```python
from build123d import *

# Parameters (mm, degrees)
F1_DEPTH     = 56.134
F3_DEPTH     = 12.7
F4_T         = 6.35
F4_T3_DEPTH  = 38.1
F4_T5_DEPTH  = 38.1
F4_T8_ANGLE  = 90.000000001
F4_T10_ANGLE = 90.000000001
F4_T12_ANGLE = 90.000000001
F4_T14_ANGLE = 90.000000001


# Not quite as in the source:
# - a shell that OpenCascade refuses in one call is made with other operations: the cavity is built on its own and cut out


with BuildPart() as f1:
    # F0 (on Top) → F1 (new body)
    with BuildSketch(Plane.XY):
        with BuildLine():
            ThreePointArc((-38.1, -12.7), (-30.6605122421, -30.6605122421), (-12.7, -38.1))
            Line((-12.7, -38.1), (12.7, -38.1))
            ThreePointArc((12.7, -38.1), (30.6605122421, -30.6605122421), (38.1, -12.7))
            Line((38.1, -12.7), (38.1, 12.7))
            ThreePointArc((38.1, 12.7), (30.6605122421, 30.6605122421), (12.7, 38.1))
            Line((12.7, 38.1), (-12.7, 38.1))
            ThreePointArc((-12.7, 38.1), (-30.6605122421, 30.6605122421), (-38.1, 12.7))
            Line((-38.1, 12.7), (-38.1, -12.7))
        make_face()
    extrude(amount=F1_DEPTH)

    # F2 (on face) → F3 (join)
    with BuildSketch(Plane.XY.offset(56.134)):
        with BuildLine():
            ThreePointArc((-50.8, -38.1), (-47.0802561211, -47.0802561211), (-38.1, -50.8))
            Line((-38.1, -50.8), (38.1, -50.8))
            ThreePointArc((38.1, -50.8), (47.0802561211, -47.0802561211), (50.8, -38.1))
            Line((50.8, -38.1), (50.8, 38.1))
            ThreePointArc((50.8, 38.1), (47.0802561211, 47.0802561211), (38.1, 50.8))
            Line((38.1, 50.8), (-38.1, 50.8))
            ThreePointArc((-38.1, 50.8), (-47.0802561211, 47.0802561211), (-50.8, 38.1))
            Line((-50.8, 38.1), (-50.8, -38.1))
        make_face()
    extrude(amount=F3_DEPTH)

    # F4: shell of thickness 6.35, made by hand


with BuildPart() as f4_core1:
    # F4_t2: copy of F1
    add(f1.part)

    # the walls: a layer under each face that stays
    f4_faces = [f4_core1.faces().sort_by_distance(p)[0] for p in [
        (-47.0802561211, -47.0802561211, 62.484),
        (-50.8, 0, 62.484),
        (0, -50.8, 62.484),
        (-33.8666666667, -33.8666666667, 56.134),
        (0, 0, 68.834),
        (-47.0802561211, 47.0802561211, 62.484),
        (47.0802561211, -47.0802561211, 62.484),
        (0, 50.8, 62.484),
        (50.8, 0, 62.484),
        (47.0802561211, 47.0802561211, 62.484),
        (-38.1, 0, 28.067),
        (-30.6605122421, -30.6605122421, 28.067),
        (0, -38.1, 28.067),
        (30.6605122421, -30.6605122421, 28.067),
        (38.1, 0, 28.067),
        (30.6605122421, 30.6605122421, 28.067),
        (0, 38.1, 28.067),
        (-30.6605122421, 30.6605122421, 28.067),
    ]]
    thicken(f4_faces, amount=-F4_T, mode=Mode.SUBTRACT)

    # F4_s4 → F4_t3 (cut)
    with BuildSketch(Plane.XZ.offset(-19.05)):
        Polygon((-38.1635, 56.0705), (-38.1, 62.484), (-31.75, 62.484), (-31.75, 56.134), align=None)
        Polygon((38.1635, 56.0705), (38.1, 62.484), (31.75, 62.484), (31.75, 56.134), align=None)
    extrude(amount=F4_T3_DEPTH, mode=Mode.SUBTRACT)

    # F4_s6 → F4_t5 (cut)
    with BuildSketch(Plane.YZ.offset(-19.05)):
        Polygon((-38.1635, 56.0705), (-38.1, 62.484), (-31.75, 62.484), (-31.75, 56.134), align=None)
        Polygon((38.1635, 56.0705), (38.1, 62.484), (31.75, 62.484), (31.75, 56.134), align=None)
    extrude(amount=F4_T5_DEPTH, mode=Mode.SUBTRACT)

    # F4_s7 → F4_t8 (revolve, cut)
    with BuildSketch(Plane.XZ.offset(12.7)):
        Polygon((-38.1635, 56.0705), (-38.1, 62.484), (-31.75, 62.484), (-31.75, 56.134), align=None)
    revolve(axis=Axis((-12.7, -12.7, 56.134), (0, 0, 1)), revolution_arc=F4_T8_ANGLE, mode=Mode.SUBTRACT)

    # F4_s9 → F4_t10 (revolve, cut)
    with BuildSketch(Plane.YZ.offset(12.7)):
        Polygon((-38.1635, 56.0705), (-38.1, 62.484), (-31.75, 62.484), (-31.75, 56.134), align=None)
    revolve(axis=Axis((12.7, -12.7, 56.134), (0, 0, 1)), revolution_arc=F4_T10_ANGLE, mode=Mode.SUBTRACT)

    # F4_s11 → F4_t12 (revolve, cut)
    with BuildSketch(Plane.XZ.offset(-12.7)):
        Polygon((38.1635, 56.0705), (38.1, 62.484), (31.75, 62.484), (31.75, 56.134), align=None)
    revolve(axis=Axis((12.7, 12.7, 56.134), (0, 0, 1)), revolution_arc=F4_T12_ANGLE, mode=Mode.SUBTRACT)

    # F4_s13 → F4_t14 (revolve, cut)
    with BuildSketch(Plane.YZ.offset(-12.7)):
        Polygon((38.1635, 56.0705), (38.1, 62.484), (31.75, 62.484), (31.75, 56.134), align=None)
    revolve(axis=Axis((-12.7, 12.7, 56.134), (0, 0, 1)), revolution_arc=F4_T14_ANGLE, mode=Mode.SUBTRACT)


with BuildPart() as f1_1:
    add(f1.part)

    # what is left inside the walls is the cavity
    f4_cavity = [f4_core1.part.solids().sort_by_distance(p)[0] for p in [
        (0, -10.583333, 62.4205),
    ]]
    add(f4_cavity, mode=Mode.SUBTRACT)


solid = f1_1.part
```
Build history of the part. All positions in model axes, mm. A direction names the side the tool comes from. Give positions to 0.01 mm unless a question says otherwise; leave off trailing zeros. Order: outer loops, then holes, each group sorted by start corner. A loop starts at its lowest first (then second) coordinate and runs counter-clockwise, first axis right, second up. Notation, with made-up numbers: M 27.25,72 L 33.25,72 A20 ccw 33.25,80 Z; hole C 78,37 d2. An arc over 180 degrees is marked long. Return JSON: item names as keys, results as strings.
Q1. 3-axis set-ups, long thin cutter, end or side, ignore diameter. For faces 4 (the face through (30.86, 30.46, 27.67)), 5 (the face through (0, 0, 62.484)), 6 (the face through (-30.86, -30.46, 27.67)): which of +Z, -Z, +X, -X, +Y, -Y reach the whole face in a straight line?
Answer list:
{"face 4": "-Z, +X, +Y", "face 5": "-Z", "face 6": "-Z, -X, -Y"}
Q2. Band-saw the part on A-A (z = 30.5). Give the cut face in (x, y), then the cut area to 3 significant figures.
Answer list:
{"outline": "M -38.1,-12.7 A25.4 ccw -12.7,-38.1 L 12.7,-38.1 A25.4 ccw 38.1,-12.7 L 38.1,12.7 A25.4 ccw 12.7,38.1 L -12.7,38.1 A25.4 ccw -38.1,12.7 Z; hole M -31.75,-12.7 A19.05 ccw -12.7,-31.75 L 12.7,-31.75 A19.05 ccw 31.75,-12.7 L 31.75,12.7 A19.05 ccw 12.7,31.75 L -12.7,31.75 A19.05 ccw -31.75,12.7 Z", "area": "1,530 mm^2"}
Q3. Band-saw the part on D-D (y = 24). Give the cut face in (x, z).
Answer list:
{"outline": "M -50.8,56.13 L -35.45,56.13 L -35.45,0 L -28.04,0 L -28.04,62.48 L 28.04,62.48 L 28.04,0 L 35.45,0 L 35.45,56.13 L 50.8,56.13 L 50.8,68.83 L -50.8,68.83 Z"}
Q4. Flat gauge pins, fed straight in: pin 1 (4 mm diameter, centred on y = 3, z = 11.5, fed in from -X); pin 2 (8 mm diameter, centred on y = 34.5, z = 22, fed in from +X); pin 3 (1.5 mm diameter, centred on x = 16.5, y = -3, fed in from -Z). Where does each tip first touch, or does it go through?
Answer list:
{"pin 1": "stops at x = -38.1", "pin 2": "stops at x = 30.82", "pin 3": "stops at z = 62.48"}
Q5. Band-saw the part on B-B (x = 0). Give the cut face in (y, z), then the cut area to 3 significant figures.
Answer list:
{"outline": "M -50.8,56.13 L -38.1,56.13 L -38.1,0 L -31.75,0 L -31.75,62.48 L 31.75,62.48 L 31.75,0 L 38.1,0 L 38.1,56.13 L 50.8,56.13 L 50.8,68.83 L -50.8,68.83 Z", "area": "1,600 mm^2"}
Q6. Wall check: probe 1 along X at (y, z) = (8.5, 27); probe 2 along Z at (x, y) = (25.5, 43.5). Give the ranges that are in metal, low to high. Write a range as from..to.
Answer list:
{"probe 1": "x = -38.1..-31.75, 31.75..38.1", "probe 2": "z = 56.13..68.83"}
Q7. Two-plate mould, pull along Y, no slides. Class faces 1 (the face through (0, 31.75, 32)), 2 (the face through (0, 38.1, 28)), 3 (the face through (-38.1, 0, 28)): pulls with the +Y half, pulls with the -Y half, needs draft (parallel to the pull), parting line crosses it, or undercut.
Answer list:
{"face 1": "undercut", "face 2": "pulls with the +Y half", "face 3": "needs draft"}
